For this review, take the finished solid that the model builds, in its own axes (mm). Coordinates: 2 decimals unless noted, no trailing zeros. Write each loop counter-clockwise with the first axis right and the second up, starting at its lowest first coordinate (ties: lowest second). Pieces come first, ordered by that corner, then holes. Notation, with made-up numbers: (26.5, -8.5) -> (61.5, -8.5) arc R20 ccw to (61.5, 24.5) -> close; hole circle Ø11 at (65, 50). An arc over 180 degrees is marked (long way). Put each result on its own line as item: value. Start each with the question number.
Item 1: Consider section D-D on x = 18. Give the boundary of the cut face in (y, z), and give its area (3 significant figures).
Item 2: To check wall thickness, follow L1, parallel to Y at x = 30, z = 1.7; L2, parallel to Y at x = 37, z = 0.6; L3, parallel to X at y = -102, z = 1.6. State the ranges of each line that lie inside material, in increasing order.
Item 3: Consider section B-B on x = 30. Give the boundary of the cut face in (y, z).
Item 4: Insertion check: P1, Ø4, axis at x = 55.1, y = -55.1, coming from the -Z side. The pin has a flat end and moves straight along its axis. Give the tip position at first contact, or say it passes through.
Item 5: Consider section A-A on y = -90. Give the boundary of the cut face in (x, z).
Item 6: Consider section C-C on z = 2. Give the boundary of the cut face in (x, y), and give its area (3 significant figures).
Item 7: The part is to be moulded in two halves that separate along X. For faces 1 (the flat face through (30, -59, 0)), 2 (the cylindrical face through (24.58, -114.406, 2.465)), 3 (the flat face through (60, -61, 2)), say which applies: +X half, -X half, draft (parallel to the pull), parting line (faces both ways), or undercut.
```python
from build123d import *

# Parameters (mm, degrees)
F0_R     = 25
F0_R_2   = 21.905378
F1_DEPTH = 5
F2_R     = 2.25
F3_DEPTH = 25


with BuildPart() as f1:
    # F0 (on Top) → F1 (new body)
    with BuildSketch(Plane.XY):
        with BuildLine():
            Line((57, 0), (3, 0))
            ThreePointArc((3, 0), (0.87868, -0.87868), (0, -3))
            Line((0, -3), (0, -117))
            ThreePointArc((0, -117), (0.87868, -119.12132), (3, -120))
            Line((3, -120), (57, -120))
            ThreePointArc((57, -120), (59.12132, -119.12132), (60, -117))
            Line((60, -117), (60, -3))
            ThreePointArc((60, -3), (59.12132, -0.87868), (57, 0))
        make_face()
        with Locations((30, -90)):
            Circle(F0_R, mode=Mode.SUBTRACT)
        with Locations((30, -28.094622)):
            Circle(F0_R_2, mode=Mode.SUBTRACT)
    extrude(amount=F1_DEPTH)

    # F2 (on face) → F3 (cut)
    with BuildSketch(Plane.XY.offset(5)):
        with Locations((4.897709, -115.102291)):
            Circle(F2_R)
        with Locations((55.102291, -64.897709)):
            Circle(F2_R)
        with Locations((55.102291, -55.102291)):
            Circle(F2_R)
        with Locations((4.897709, -4.897709)):
            Circle(F2_R)
    extrude(amount=-F3_DEPTH, mode=Mode.SUBTRACT)


solid = f1.part
```
Return value:
1. outline: (-120, 0) -> (-111.93, 0) -> (-111.93, 5) -> (-120, 5) -> close; (-68.07, 0) -> (-46.42, 0) -> (-46.42, 5) -> (-68.07, 5) -> close; (-9.77, 0) -> (0, 0) -> (0, 5) -> (-9.77, 5) -> close
1. area: 197 mm^2
2. L1: -120 to -115, -65 to -50, -6.19 to 0
2. L2: -120 to -114, -66 to -48.85, -7.34 to 0
2. L3: 0 to 8.07, 51.93 to 60
3. outline: (-120, 0) -> (-115, 0) -> (-115, 5) -> (-120, 5) -> close; (-65, 0) -> (-50, 0) -> (-50, 5) -> (-65, 5) -> close; (-6.19, 0) -> (0, 0) -> (0, 5) -> (-6.19, 5) -> close
4. P1: through
5. outline: (0, 0) -> (5, 0) -> (5, 5) -> (0, 5) -> close; (55, 0) -> (60, 0) -> (60, 5) -> (55, 5) -> close
6. outline: (0, -117) arc R3 ccw to (3, -120) -> (57, -120) arc R3 ccw to (60, -117) -> (60, -3) arc R3 ccw to (57, 0) -> (3, 0) arc R3 ccw to (0, -3) -> close; hole circle Ø4.5 at (4.9, -115.1); hole circle Ø4.5 at (4.9, -4.9); hole circle Ø50 at (30, -90); hole circle Ø43.81 at (30, -28.09); hole circle Ø4.5 at (55.1, -64.9); hole circle Ø4.5 at (55.1, -55.1)
6. area: 3,660 mm^2
7. face 1: draft
7. face 2: undercut
7. face 3: +X half
